Geometry check sheet. Reference: the model listing, model coordinates, mm. Give positions to 0.01 mm unless a question says otherwise; leave off trailing zeros. Order: outer loops, then holes, each group sorted by start corner. A loop starts at its lowest first (then second) coordinate and runs counter-clockwise, first axis right, second up. Notation, with made-up numbers: (7.25, 26.25) - (54.25, 26.25) arc R24 cw to (54.25, 63.25) - close; hole circle Ø4 at (-36, 11). An arc over 180 degrees is marked (long way). Put each result on its own line as item: value. Start each with the question number.
```python
from build123d import *

# Parameters (mm, degrees)
SKETCH1_R               = 11
SKETCH1_R_2             = 4
BOSS_EXTRUDE1_DEPTH     = 6.35
CUT_EXTRUDE1_DEPTH      = 380.972155331
CUT_EXTRUDE1_DEPTH_BACK = 380.972155331
SKETCH2_R               = 6.35


with BuildPart() as part:
    # Sketch1 → Boss-Extrude1 (new body)
    with BuildSketch(Plane.XY):
        with BuildLine():
            ThreePointArc((-14.847301451, 14.171565356), (-18.06169524, -9.749399473), (3.699835438, -20.18878012))
            ThreePointArc((3.699835438, -20.18878012), (74.556998508, -9.322867247), (145.926048807, -2.594993863))
            ThreePointArc((145.926048807, -2.594993863), (251.652155026, -1.855156614), (356.755502219, -13.337460579))
            ThreePointArc((356.755502219, -13.337460579), (371.894318042, -4.08193425), (364.839650306, 12.199348725))
            ThreePointArc((364.839650306, 12.199348725), (258.044932978, 52.392610297), (145.926048807, 73.605006137))
            ThreePointArc((145.926048807, 73.605006137), (58.666161858, 62.481005213), (-14.847301451, 14.171565356))
        make_face()
        Circle(SKETCH1_R, mode=Mode.SUBTRACT)
        with Locations((359, 0)):
            Circle(SKETCH1_R_2, mode=Mode.SUBTRACT)
    extrude(amount=BOSS_EXTRUDE1_DEPTH)

    # Sketch2 → Cut-Extrude1 (cut, two sides: drawn at the far end of the back side and taken through both)
    with BuildSketch(Plane.XY.offset(6.35).offset(-CUT_EXTRUDE1_DEPTH_BACK)):
        with Locations((32.051371855, 20.599018477)):
            Circle(SKETCH2_R)
    extrude(amount=CUT_EXTRUDE1_DEPTH + CUT_EXTRUDE1_DEPTH_BACK, mode=Mode.SUBTRACT)


solid = part.part
```
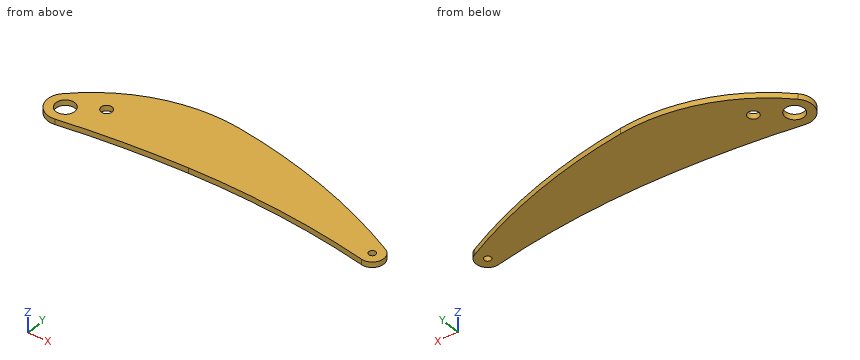
Item 1: Thickness scan on line 1 along Y through (x, z) = (359, 4.75) (3 decimals); line 2 along Y through (x, z) = (0, 1.5) (3 decimals); line 3 along Y through (x, z) = (161, 5.75). Record the ranges inside material, lowest first.
Item 2: Cross-section at A-A (x = 0). Enter the section's corners in (y, z) (3 decimals), and give its area (3 significant figures).
Item 3: Cross-section at D-D (x = 117). Enter the section's corners in (y, z), and give its area (3 significant figures).
Item 4: Gauge pin test, flat ends, axial feed: pin 1 Ø1 at (y, z) = (-7, 3) entering from +X; pin 2 Ø7.5 at (x, y) = (32.05, 20.6) entering from -Z; pin 3 Ø2 at (x, z) = (212, 1.5) entering from +Y; pin 4 Ø1 at (y, z) = (11.5, 1) entering from +X. Record the tip position at first contact, or that the pin passes through.
Item 5: Cross-section at B-B (z = 4.25). Count the separate pieces of the cut face and the enclosed holes in it, and give its area (3 significant figures).
Item 6: Cross-section at C-C (y = 42). Enter the section's corners in (x, z), and give its area (3 significant figures).
Recorded:
1. line 1: y = -13.525 to -4, 4 to 14.96
1. line 2: y = -20.525 to -11, 11 to 28.181
1. line 3: y = -1.74 to 71.91
2. outline: (-20.525, 0) - (-11, 0) - (-11, 6.35) - (-20.525, 6.35) - close; (11, 0) - (28.181, 0) - (28.181, 6.35) - (11, 6.35) - close
2. area: 170 mm^2
3. outline: (-4.82, 0) - (74.37, 0) - (74.37, 6.35) - (-4.82, 6.35) - close
3. area: 503 mm^2
4. pin 1: stops at x = 370.86
4. pin 2: passes through
4. pin 3: stops at y = 63.75
4. pin 4: stops at x = 366.87
5. separate pieces: 1
5. enclosed holes: 3
5. area: 22,600 mm^2
6. outline: (18.36, 0) - (291.63, 0) - (291.63, 6.35) - (18.36, 6.35) - close
6. area: 1,740 mm^2
